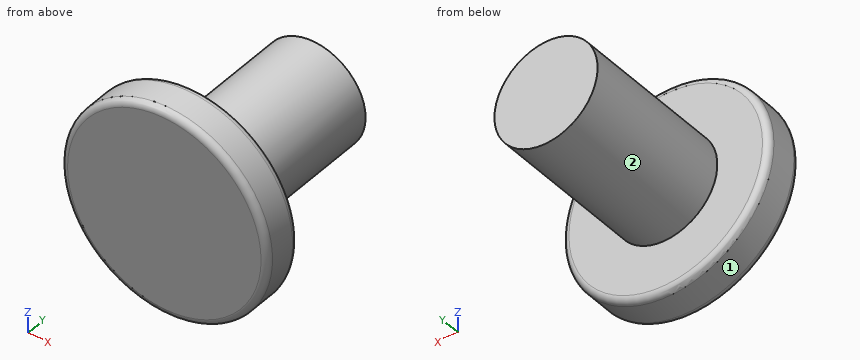
Autodesk Inventor part; units mm, degrees
ref_plane "YZ Plane" through (0, 0, 0) normal (1, 0, 0) x (0, 1, 0)
ref_plane "XZ Plane" through (0, 0, 0) normal (0, 1, 0) x (-1, 0, 0)
ref_plane "XY Plane" through (0, 0, 0) normal (0, 0, 1) x (1, 0, 0)
sketch "Sketch1" plane through (0, 0, 0) normal (0, 1, 0) x (-1, 0, 0)
  circle A0 centre (0, 0) radius 8
  dimension "d0" = 16
extrude "Extrusion1" add sketch "Sketch1" along normal blind 3
sketch "Sketch2" plane through (0, 3, 0) normal (0, 1, 0) x (1, 0, 0)
  circle A0 centre (0, 0) radius 4
  dimension "d3" = 8
extrude "Extrusion2" add sketch "Sketch2" along normal blind 12
fillet "Fillet1" radius 0.5 2 edges at (8, 3, 0) (8, 0, 0)
thread "Thread2"
properties part number "M3_12mm"
The listing builds one solid part. Answer for the finished solid, in the listing's coordinates (mm). Face numbers are marked on the shaded views. A direction names the side the tool comes from. Give positions to 0.01 mm unless a question says otherwise; leave off trailing zeros. Write each loop counter-clockwise with the first axis right and the second up, starting at its lowest first coordinate (ties: lowest second). Pieces come first, ordered by that corner, then holes. Notation, with made-up numbers: (29, 81) -> (75, 81) arc R18 cw to (75, 86) -> close; hole circle Ø1 at (58.5, 34.25). An arc over 180 degrees is marked (long way). One line per question, with ' | ' between items. Start each with the question number.
1. Section B-B (x = 0) is taken. Determine the outline of the cut face in (y, z).
2. For the marked faces 1 and 2, determine the directions among +Z, -Z, +X, -X, +Y, -Y from which every point of the face is accessible in a straight line to the end or side of a thin tool.
3. Section D-D (y = 9) is taken. Determine the outline of the cut face in (x, z).
4. Section A-A (z = 0) is taken. Determine the outline of the cut face in (x, y), plus the area to 3 significant figures.
5. Find the intervals of material crossed by probe 1 along Y at (x, z) = (-2.75, 3.75); probe 2 along Z at (x, y) = (2.5, 10); probe 3 along X at (y, z) = (9.5, -1), in increasing order.
6. Given pin 1 Ø2 at (y, z) = (7, -3) entering from +X; pin 2 Ø5 at (x, y) = (-2, 6) entering from -Z; pin 3 Ø8 at (x, z) = (-4.5, -2.5) entering from +Y; pin 4 Ø6 at (y, z) = (10, 0.5) entering from +X, each flat-ended and moving along its own axis, determine where each tip first touches the part or whether it passes through.
7. Section C-C (y = 1) is taken. Determine the outline of the cut face in (x, z), plus the area to 3 significant figures.
Response values:
1) outline: (0, -7.5) arc R0.5 ccw to (0.5, -8) -> (2.5, -8) arc R0.5 ccw to (3, -7.5) -> (3, -4) -> (15, -4) -> (15, 4) -> (3, 4) -> (3, 7.5) arc R0.5 ccw to (2.5, 8) -> (0.5, 8) arc R0.5 ccw to (0, 7.5) -> close
2) face 1: +Y, -Y | face 2: +Y
3) outline: circle Ø8 at (0, 0)
4) outline: (-8, 0.5) arc R0.5 ccw to (-7.5, 0) -> (7.5, 0) arc R0.5 ccw to (8, 0.5) -> (8, 2.5) arc R0.5 ccw to (7.5, 3) -> (4, 3) -> (4, 15) -> (-4, 15) -> (-4, 3) -> (-7.5, 3) arc R0.5 ccw to (-8, 2.5) -> close | area: 144 mm2
5) probe 1: 0 to 3 | probe 2: -3.12 to 3.12 | probe 3: -3.87 to 3.87
6) pin 1: x = 3.46 | pin 2: z = -4 | pin 3: y = 15 | pin 4: x = 4
7) outline: circle Ø16 at (0, 0) | area: 201 mm2
